Geometry check sheet. Reference: the model listing, model coordinates, mm. A direction names the side the tool comes from. Coordinates: 2 decimals unless noted, no trailing zeros. Write each loop counter-clockwise with the first axis right and the second up, starting at its lowest first coordinate (ties: lowest second). Pieces come first, ordered by that corner, then holes. Notation, with made-up numbers: (19, -27.75) -> (35, -27.75) arc R22 cw to (35, -12.75) -> close; hole circle Ø2 at (3.25, 2). An arc over 180 degrees is marked (long way). Use a Markdown table: item, result.
```python
from build123d import *

# Parameters (mm, degrees)
SKETCH1_W           = 39.878
SKETCH1_H           = 18.796
BOSS_EXTRUDE1_DEPTH = 39.878
SKETCH2_W           = 18.796
SKETCH2_H           = 2.794
BOSS_EXTRUDE2_DEPTH = 7.493
SKETCH3_W           = 18.796
SKETCH3_H           = 2.794
BOSS_EXTRUDE3_DEPTH = 7.493
SKETCH6_R           = 3.908083023
BOSS_EXTRUDE5_DEPTH = 5.08
SKETCH7_R           = 3.048
CUT_EXTRUDE1_DEPTH  = 5.08


with BuildPart() as part:
    # Sketch1 → Boss-Extrude1 (new body)
    with BuildSketch(Plane(origin=(0, 0, 0), x_dir=(1, 0, 0), z_dir=(0, 1, 0))):
        with Locations((19.939, 9.398)):
            Rectangle(SKETCH1_W, SKETCH1_H)
    extrude(amount=BOSS_EXTRUDE1_DEPTH)

    # Sketch2 → Boss-Extrude2 (add)
    with BuildSketch(Plane.ZY):
        with Locations((-9.398, 29.337)):
            Rectangle(SKETCH2_W, SKETCH2_H)
    extrude(amount=BOSS_EXTRUDE2_DEPTH)

    # Sketch3 → Boss-Extrude3 (add)
    with BuildSketch(Plane(origin=(39.878, 0, 0), x_dir=(0, 0, -1), z_dir=(1, 0, 0))):
        with Locations((9.398, 29.337)):
            Rectangle(SKETCH3_W, SKETCH3_H)
    extrude(amount=BOSS_EXTRUDE3_DEPTH)

    # Sketch6 → Boss-Extrude5 (add)
    with BuildSketch(Plane(origin=(0, 39.878, 0), x_dir=(1, 0, 0), z_dir=(0, 1, 0))):
        with Locations(Location((8.89, 9.764757061, 0), (0, 0, 90))):
            Circle(SKETCH6_R)
    extrude(amount=BOSS_EXTRUDE5_DEPTH)

    # Sketch7 → Cut-Extrude1 (cut)
    with BuildSketch(Plane(origin=(0, 30.734, 0), x_dir=(1, 0, 0), z_dir=(0, 1, 0))):
        with Locations((-4.471485828, 14.097)):
            Circle(SKETCH7_R)
        with Locations((-4.471485828, 4.699)):
            Circle(SKETCH7_R)
        with Locations((44.349485828, 4.699)):
            Circle(SKETCH7_R)
        with Locations((44.349485828, 14.097)):
            Circle(SKETCH7_R)
    extrude(amount=-CUT_EXTRUDE1_DEPTH, mode=Mode.SUBTRACT)


solid = part.part
```
Item 1: Section check A-A on x = 8.89. Record the boundary of the cut face in (y, z), then the cut area to 3 significant figures.
Answer block:
| item | result |
|---|---|
| outline | (0, -18.8) -> (39.88, -18.8) -> (39.88, -13.67) -> (44.96, -13.67) -> (44.96, -5.86) -> (39.88, -5.86) -> (39.88, 0) -> (0, 0) -> close |
| area | 789 mm^2 |
Item 2: Section check D-D on z = -2.75. Record the boundary of the cut face in (x, y), then the cut area to 3 significant figures.
Answer block:
| item | result |
|---|---|
| outline | (-7.49, 27.94) -> (-6.81, 27.94) -> (-6.81, 30.73) -> (-7.49, 30.73) -> close; (-2.13, 27.94) -> (0, 27.94) -> (0, 0) -> (39.88, 0) -> (39.88, 27.94) -> (42.01, 27.94) -> (42.01, 30.73) -> (39.88, 30.73) -> (39.88, 39.88) -> (0, 39.88) -> (0, 30.73) -> (-2.13, 30.73) -> close; (46.69, 27.94) -> (47.37, 27.94) -> (47.37, 30.73) -> (46.69, 30.73) -> close |
| area | 1,610 mm^2 |
Item 3: Section check C-C on y = 24.5. Record the boundary of the cut face in (x, z).
Answer block:
| item | result |
|---|---|
| outline | (0, -18.8) -> (39.88, -18.8) -> (39.88, 0) -> (0, 0) -> close |
Item 4: Section check B-B on z = -16. Record the boundary of the cut face in (x, y).
Answer block:
| item | result |
|---|---|
| outline | (-7.49, 27.94) -> (-6.85, 27.94) -> (-6.85, 30.73) -> (-7.49, 30.73) -> close; (-2.09, 27.94) -> (0, 27.94) -> (0, 0) -> (39.88, 0) -> (39.88, 27.94) -> (41.97, 27.94) -> (41.97, 30.73) -> (39.88, 30.73) -> (39.88, 39.88) -> (0, 39.88) -> (0, 30.73) -> (-2.09, 30.73) -> close; (46.73, 27.94) -> (47.37, 27.94) -> (47.37, 30.73) -> (46.73, 30.73) -> close |
Item 5: Depth check by flat-ended pin: P1, Ø4, axis at y = 6, z = -3.5, coming from the +X side; P2, Ø5.5, axis at x = 26.5, z = -5.5, coming from the +Y side; P3, Ø3.5, axis at x = 43, z = -13, coming from the +Y side. Enter the tip coordinate at first touch or a pass-through.
Answer block:
| item | result |
|---|---|
| P1 | stops at x = 39.88 |
| P2 | stops at y = 39.88 |
| P3 | stops at y = 30.73 |
Item 6: Mould release check, pull along Z, two halves, no side actions. Record for faces 1 (the flat face through (20, 20, -18.796)), 2 (the cylindrical face through (41.304, 29.357, -14.225)), 3 (the flat face through (-7.493, 29, -2)), 4 (the flat face through (20, 20, 0)): +Z half, -Z half, draft (parallel to the pull), parting line (faces both ways), or undercut.
Answer block:
| item | result |
|---|---|
| face 1 | -Z half |
| face 2 | undercut |
| face 3 | draft |
| face 4 | +Z half |
Item 7: Tool access check on faces 5 (the flat face through (47.371, 29, -17)), 6 (the flat face through (-3, 30.734, -10)), 7 (the flat face through (0, 14, -9)), 8 (the flat face through (43, 30.734, -9)), 9 (the flat face through (43, 27.94, -9)). Record the directions out of +Z, -Z, +X, -X, +Y, -Y that give a thin tool (end or side, any length) a straight path to the whole face; none if there is none.
Answer block:
| item | result |
|---|---|
| face 5 | +Z, -Z, +X, +Y, -Y |
| face 6 | +Z, -Z, -X, +Y |
| face 7 | +Z, -Z, -X, -Y |
| face 8 | +Z, -Z, +X, +Y |
| face 9 | +Z, -Z, +X, -Y |
Item 8: Thickness scan on L1, parallel to Y at x = 11, z = -5; L2, parallel to Y at x = 41.5, z = -10.25. Record the ranges inside material, lowest first. Write a range as [from, to].
Answer block:
| item | result |
|---|---|
| L1 | y = [0, 39.88] |
| L2 | y = [27.94, 30.73] |
